Here's the drawing with two shaded views (mm, measured from the low corner). I have some questions. A direction names the side the tool comes from. Round coordinates to 2 decimals unless told otherwise and drop trailing zeros. Loops run counter-clockwise (first coordinate to the right, second up) from the corner with the lowest first, then second, coordinate; pieces in that order, holes last. Notation, with made-up numbers: M -34,-21.5 L 8,-21.5 A12 ccw 8,-11.5 Z; hole C -26,-16.75 d8. An arc over 180 degrees is marked long. Answer as a JSON object with one key per item and string values.
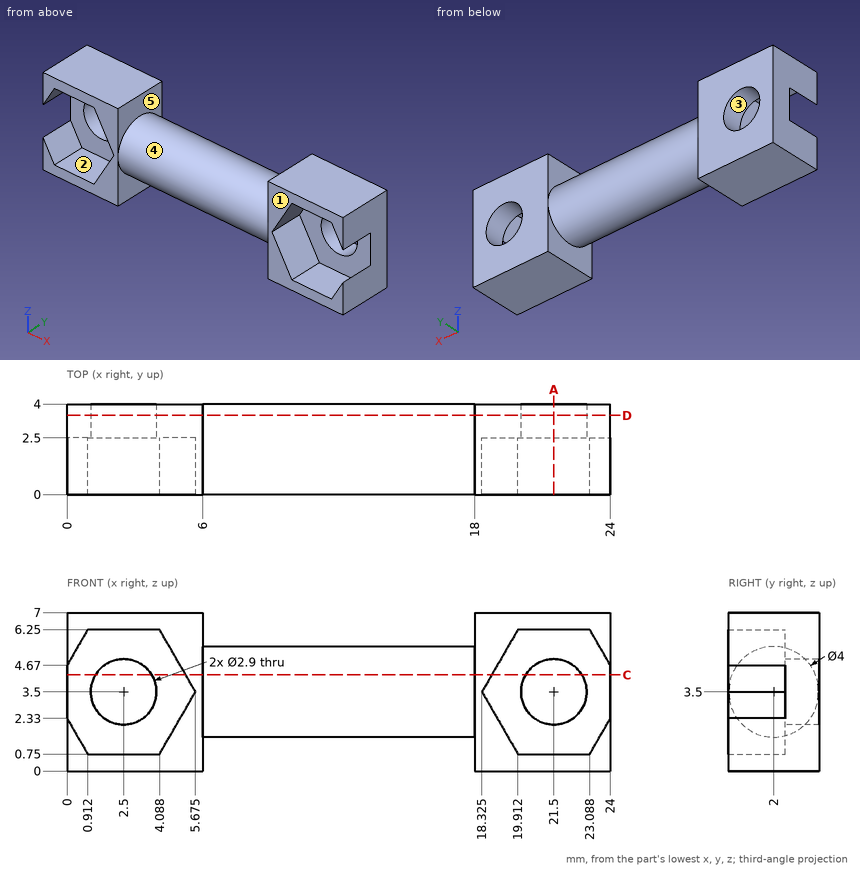
Item 1: If I drill on L1, parallel to X at y = 3.45, z = 3.5; L2, parallel to Z at x = 21.5, y = 2.9; L3, parallel to X at y = 2.9, z = 4.75 (1 decimal), over which ranges is the centre line in solid material (lowest first)? Write a range as from..to.
Solution:
{"L1": "x = 0..1.05, 3.95..20.05, 22.95..24", "L2": "z = 0..2.05, 4.95..7", "L3": "x = 0..1.8, 3.2..20.8, 22.2..24"}
Item 2: I want a section at D-D on y = 3.5. List the corners of the cut face in (x, z) for me.
Solution:
{"outline": "M 0,0 L 6,0 L 6,2.18 L 18,2.18 L 18,0 L 24,0 L 24,7 L 18,7 L 18,4.82 L 6,4.82 L 6,7 L 0,7 Z; hole C 2.5,3.5 d2.9; hole C 21.5,3.5 d2.9"}
Item 3: I want a section at C-C on z = 4.25. List the corners of the cut face in (x, y) for me.
Solution:
{"outline": "M 0,2.5 L 1.26,2.5 L 1.26,4 L 0,4 Z; M 3.74,2.5 L 5.24,2.5 L 5.24,0 L 6,0 L 6,0.15 L 18,0.15 L 18,0 L 18.76,0 L 18.76,2.5 L 20.26,2.5 L 20.26,4 L 18,4 L 18,3.85 L 6,3.85 L 6,4 L 3.74,4 Z; M 22.74,2.5 L 24,2.5 L 24,4 L 22.74,4 Z"}
Item 4: For the marked faces 1 and 2, which set-ups out of +Z, -Z, +X, -X, +Y, -Y let a thin tool reach every point of the face, with its end or its side?
Solution:
{"face 1": "+Z, -Z, +X, -X, -Y", "face 2": "-Y"}
Item 5: I want a section at A-A on x = 21.5. List the corners of the cut face in (y, z) for me.
Solution:
{"outline": "M 0,0 L 4,0 L 4,2.05 L 2.5,2.05 L 2.5,0.75 L 0,0.75 Z; M 0,6.25 L 2.5,6.25 L 2.5,4.95 L 4,4.95 L 4,7 L 0,7 Z"}
Item 6: For P1, Ø2, axis at x = 3, y = 1, coming from the -Z side; P2, Ø3, axis at x = 2.5, z = 4, coming from the -Y side; P3, Ø1, axis at x = 7, z = 4.5, coming from the -Y side, each with a flat end and sliding along its axis, tell me the tip position at first contact or that it passes through.
Solution:
{"P1": "stops at z = 0", "P2": "stops at y = 2.5", "P3": "stops at y = 0.06"}
Item 7: We'd pull the mould along Z, two halves only. Please class the marked faces 3, 4 and 5: +Z half, -Z half, draft (parallel to the pull), parting line (faces both ways), or undercut.
Solution:
{"face 3": "undercut", "face 4": "parting line", "face 5": "draft"}
